Can you work these out from the drawing? Everything is in mm from the part's minimum corner. A direction names the side the tool comes from. Give positions to 0.01 mm unless a question says otherwise; leave off trailing zeros. Order: outer loops, then holes, each group sorted by start corner. A loop starts at its lowest first (then second) coordinate and runs counter-clockwise, first axis right, second up. Notation, with made-up numbers: (-15.75, 4.5) -> (35.25, 4.5) arc R23 cw to (35.25, 18.5) -> close; hole circle Ø6 at (56.25, -15.75). An arc over 180 degrees is marked (long way). Answer as CSV lines item,"result". Start each with the question number.
(1) We'd pull the mould along Y, two halves only. Please class the marked faces 1, 2 and 3: released by +Y, released by -Y, zero draft, split by the parting line, or undercut.
(2) I need wall thicknesses on L1, parallel to X at y = 0.2, z = 5; L2, parallel to X at y = 1.55, z = 5; L3, parallel to X at y = 2.6, z = 4.5. Which ranges of each line are inside material? Lowest first, please.
(3) I want a section at B-B (y = 2.7). Please give me the cut outline in (x, z).
(4) I want a section at D-D (y = 1.8). Please give me the cut outline in (x, z), plus the area to 3 significant figures.
(5) On a 3-axis mill with a long thin cutter (end or side, diameter ignored), from which of +Z, -Z, +X, -X, +Y, -Y can I reach the whole of each face in a straight line? I mean the marked faces 4, 5 and 6. Say none if no direction works.
(6) Will this pin go through, and if not, where does the flat tip stop? pin 1 Ø6 at (x, z) = (5.5, 5) entering from -Y.
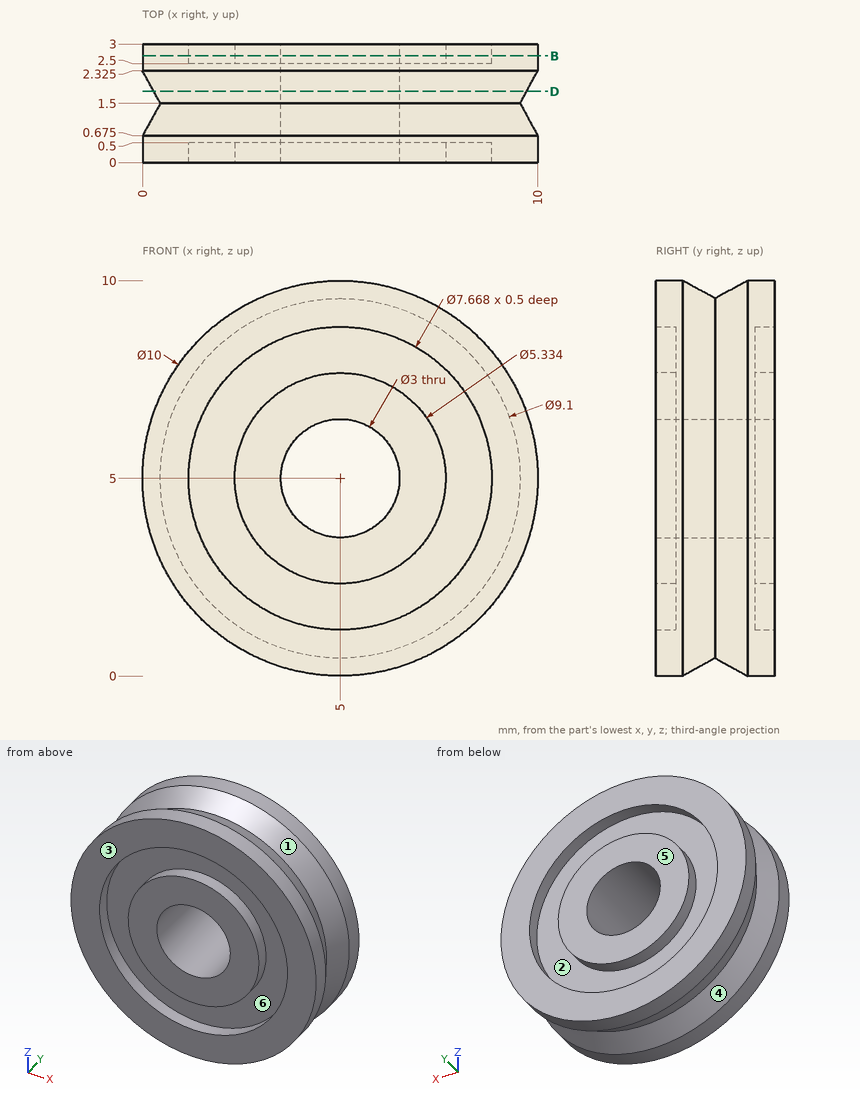
Final values:
1,face 1,"undercut"
1,face 2,"released by +Y"
1,face 3,"released by -Y"
2,L1,"0 to 1.17, 2.33 to 3.5, 6.5 to 7.67, 8.83 to 10"
2,L2,"0.42 to 3.5, 6.5 to 9.58"
2,L3,"0.03 to 1.2, 2.38 to 3.59, 6.41 to 7.62, 8.8 to 9.97"
3,outline,"circle Ø10 at (5, 5); circle Ø5.33 at (5, 5); hole circle Ø7.67 at (5, 5); hole circle Ø3 at (5, 5)"
4,outline,"circle Ø9.43 at (5, 5); hole circle Ø3 at (5, 5)"
4,area,"62.7 mm²"
5,face 4,"none"
5,face 5,"+Z, -Z, +X, -X, +Y"
5,face 6,"-Y"
6,pin 1,"y = 0"
